```python
from build123d import *

# Parameters (mm, degrees)
F0_W     = 56.269944
F0_H     = 38.358275
F1_DEPTH = 40.64
F2_R     = 15.686232
F3_DEPTH = 40.641


with BuildPart() as f1:
    # F0 (on Front) → F1 (new body)
    with BuildSketch(Plane.XZ):
        with Locations((28.134972, 19.179137)):
            Rectangle(F0_W, F0_H)
    extrude(amount=F1_DEPTH)

    # F2 (on Front) → F3 (cut, through all)
    with BuildSketch(Plane.XZ):
        with Locations((28.629173, 18.580522)):
            Circle(F2_R)
    extrude(amount=F3_DEPTH, mode=Mode.SUBTRACT)


solid = f1.part
```
Verification items for the finished model (mm, model axes). Coordinates: 2 decimals unless noted, no trailing zeros. Order: outer loops, then holes, each group sorted by start corner. A loop starts at its lowest first (then second) coordinate and runs counter-clockwise, first axis right, second up. Notation, with made-up numbers: (51.5, 55.5) -> (102.5, 55.5) arc R34 cw to (102.5, 91.5) -> close; hole circle Ø11 at (82.25, -15.75). An arc over 180 degrees is marked (long way). Put each result on its own line as item: value. Start each with the question number.
1) Cross-section at C-C (y = -19.5). Enter the section's corners in (x, z), plus the area to 3 significant figures.
2) Cross-section at A-A (z = 12). Enter the section's corners in (x, y), plus the area to 3 significant figures.
3) Release check for a two-part mould opening along X. For faces 1 (the cylindrical face through (35.867, -20.036, 4.664)), 2 (the flat face through (56.27, -20, 19)), 3 (the flat face through (28, -20, 0)) record: pulls with the +X half, pulls with the -X half, needs draft (parallel to the pull), parting line crosses it, or undercut.
4) Cross-section at B-B (x = 29.5). Enter the section's corners in (y, z).
5) Material ranges on L1, parallel to X at y = -25.5, z = 18.5; L2, parallel to Z at x = 27, y = -35; L3, parallel to X at y = -31, z = 22, recorded low to high.
6) Go/stop test with a flat-tipped pin: pin 1 (8 mm diameter, centred on x = 19.5, z = 24.5, fed in from +Y). Record where the tip stops, or that it passes through.
Geometry check:
1. outline: (0, 0) -> (56.27, 0) -> (56.27, 38.36) -> (0, 38.36) -> close; hole circle Ø31.37 at (28.63, 18.58)
1. area: 1,390 mm^2
2. outline: (0, -40.64) -> (14.39, -40.64) -> (14.39, 0) -> (0, 0) -> close; (42.87, -40.64) -> (56.27, -40.64) -> (56.27, 0) -> (42.87, 0) -> close
2. area: 1,130 mm^2
3. face 1: undercut
3. face 2: pulls with the +X half
3. face 3: needs draft
4. outline: (-40.64, 0) -> (0, 0) -> (0, 2.92) -> (-40.64, 2.92) -> close; (-40.64, 34.24) -> (0, 34.24) -> (0, 38.36) -> (-40.64, 38.36) -> close
5. L1: x = 0 to 12.94, 44.32 to 56.27
5. L2: z = 0 to 2.98, 34.18 to 38.36
5. L3: x = 0 to 13.32, 43.94 to 56.27
6. pin 1: passes through
